Could you check a few things on this model? Use its own coordinates, in mm. Round coordinates to 2 decimals unless told otherwise and drop trailing zeros. Write each loop counter-clockwise with the first axis right and the second up, starting at its lowest first coordinate (ties: lowest second). Pieces come first, ordered by that corner, then holes.
```python
from build123d import *

# Parameters (mm, degrees)
F0_W        = 38
F0_H        = 8
F0_R        = 2.5
F1_DEPTH    = 8
F2_T1_DEPTH = 28.32


# Not quite as in the source:
# - a fillet or chamfer that OpenCascade refuses, or shapes differently, is made with other operations: its cross-section is extruded or revolved along the edge and cut away or added


with BuildPart() as f1:
    # F0 (on Top) → F1 (new body)
    with BuildSketch(Plane.XY):
        Rectangle(F0_W, F0_H)
        with BuildLine():
            ThreePointArc((-18.5, 0), (-16, 2.5), (-13.5, 0))
            ThreePointArc((-13.5, 0), (-16, -2.5), (-18.5, 0))
        make_face(mode=Mode.SUBTRACT)
        with Locations((-8, 0)):
            Circle(F0_R, mode=Mode.SUBTRACT)
        Circle(F0_R, mode=Mode.SUBTRACT)
        with Locations((8, 0)):
            Circle(F0_R, mode=Mode.SUBTRACT)
        with Locations((16, 0)):
            Circle(F0_R, mode=Mode.SUBTRACT)
    extrude(amount=F1_DEPTH)

    # F2: fillet of radius 4.064 on 4 edges, made by hand

    # F2_s2 → F2_t1 (cut)
    with BuildSketch(Plane.XY.offset(-10.16)):
        with BuildLine():
            ThreePointArc((14.936, -4), (17.8096819587, -2.8096819587), (19, 0.064))
            Line((19, 0.064), (19, -4))
            Line((19, -4), (14.936, -4))
        make_face()
        with BuildLine():
            ThreePointArc((14.936, 4), (17.8096819587, 2.8096819587), (19, -0.064))
            Line((19, -0.064), (19, 4))
            Line((19, 4), (14.936, 4))
        make_face()
        with BuildLine():
            ThreePointArc((-14.936, -4), (-17.8096819587, -2.8096819587), (-19, 0.064))
            Line((-19, 0.064), (-19, -4))
            Line((-19, -4), (-14.936, -4))
        make_face()
        with BuildLine():
            ThreePointArc((-14.936, 4), (-17.8096819587, 2.8096819587), (-19, -0.064))
            Line((-19, -0.064), (-19, 4))
            Line((-19, 4), (-14.936, 4))
        make_face()
    extrude(amount=F2_T1_DEPTH, mode=Mode.SUBTRACT)


solid = f1.part
```
Q1. Imagine slicing it at A-A, the plane z = 0.75. Write out the boundary of the cut face in (x, y), then the cut area to 3 significant figures.
Q2. If I drill on L1, parallel to Y at x = 8, z = 4; L2, parallel to X at y = -0.75, z = 2.25; L3, parallel to X at y = -0.5, z = 5, over which ranges is the centre line in solid material (lowest first)?
Q3. Imagine slicing it at C-C, the plane y = -1.25. Write out the boundary of the cut face in (x, z), then the cut area to 3 significant figures.
Q4. I'm going to push a flat-ended pin straight in: pin 1 Ø4 at (x, y) = (16, 0) entering from -Z. Where does the tip first touch, or does it pass through?
Q5. Imagine slicing it at B-B, the plane x = -8. Write out the boundary of the cut face in (y, z), then the cut area to 3 significant figures.
Q6. We'd pull the mould along X, two halves only. Please class faces 1 (the cylindrical face through (17.76, 2.86, 3.94)), 2 (the flat face through (0, 3, 0)), 3 (the cylindrical face through (13.5, 0.1, 3.9)): pulls with the +X half, pulls with the -X half, needs draft (parallel to the pull), parting line crosses it, or undercut.
Q7. Imagine slicing it at D-D, the plane x = 2. Write out the boundary of the cut face in (y, z).
Results found:
1. outline: (-19, 0) arc R4.06 ccw to (-14.94, -4) - (14.94, -4) arc R4.06 ccw to (19, 0) arc R4.06 ccw to (14.94, 4) - (-14.94, 4) arc R4.06 ccw to start; hole circle Ø5 at (-16, 0); hole circle Ø5 at (-8, 0); hole circle Ø5 at (0, 0); hole circle Ø5 at (8, 0); hole circle Ø5 at (16, 0)
1. area: 192 mm2
2. L1: y = -4 to -2.5, 2.5 to 4
2. L2: x = -18.92 to -18.38, -13.62 to -10.38, -5.62 to -2.38, 2.38 to 5.62, 10.38 to 13.62, 18.38 to 18.92
2. L3: x = -18.96 to -18.45, -13.55 to -10.45, -5.55 to -2.45, 2.45 to 5.55, 10.45 to 13.55, 18.45 to 18.96
3. outline: (-18.78, 0) - (-18.17, 0) - (-18.17, 8) - (-18.78, 8) - close; (-13.83, 0) - (-10.17, 0) - (-10.17, 8) - (-13.83, 8) - close; (-5.83, 0) - (-2.17, 0) - (-2.17, 8) - (-5.83, 8) - close; (2.17, 0) - (5.83, 0) - (5.83, 8) - (2.17, 8) - close; (10.17, 0) - (13.83, 0) - (13.83, 8) - (10.17, 8) - close; (18.17, 0) - (18.78, 0) - (18.78, 8) - (18.17, 8) - close
3. area: 127 mm2
4. pin 1: passes through
5. outline: (-4, 0) - (-2.5, 0) - (-2.5, 8) - (-4, 8) - close; (2.5, 0) - (4, 0) - (4, 8) - (2.5, 8) - close
5. area: 24.0 mm2
6. face 1: pulls with the +X half
6. face 2: needs draft
6. face 3: undercut
7. outline: (-4, 0) - (-1.5, 0) - (-1.5, 8) - (-4, 8) - close; (1.5, 0) - (4, 0) - (4, 8) - (1.5, 8) - close
